Geometry: final body of the model. Coordinates: model frame, mm. Give positions to 0.01 mm unless a question says otherwise; leave off trailing zeros. Loops run counter-clockwise (first coordinate to the right, second up) from the corner with the lowest first, then second, coordinate; pieces in that order, holes last. Notation, with made-up numbers: (7.25, 31.5) -> (13.25, 31.5) arc R11 cw to (13.25, 48.5) -> close; hole circle Ø11 at (75.5, 1.25). An arc over 180 degrees is marked (long way). One line per question, with ' | ' between items. Start each with the question number.
Item 1: Section D-D on x = 35.5. Return loops of the section in (y, z) (3 decimals).
Item 2: Pin query (flat end, axial travel): P1, Ø3, axis at x = 33, y = -23.5, coming from the +Z side. Return the tip coordinate at first contact, or that it passes through.
Item 3: Material intervals for line 1 along Z through (x, y) = (22, -20); line 2 along Y through (x, z) = (26, 43); line 3 along Z through (x, y) = (41, -22), sorted ascending. Write a range as [from, to].
Item 4: Section A-A on x = 7. Return loops of the section in (y, z) (3 decimals), then the cut area to 3 significant figures.
Item 5: Section C-C on x = 26.7. Return loops of the section in (y, z) (3 decimals).
Item 6: Section B-B on z = 22. Return loops of the section in (x, y) (3 decimals).
Item 7: Mould query, pull axis Y, two halves, no side actions, for faces 1 (the flat face through (27, 0, 43.675)), 2 (the flat face through (16, 0, 43.875)), 3 (the cylindrical face through (16.76, -26.67, 41.02)). Classes: released by +Y, released by -Y, zero draft, split by the parting line, or undercut.
from build123d import *

# Parameters (mm, degrees)
SKETCH1_W           = 87.75
SKETCH1_H           = 59.35
BOSS_EXTRUDE1_DEPTH = 43.05
FILLET1_R           = 10
SKETCH2_R           = 4.3
CUT_EXTRUDE1_DEPTH  = 0.2


with BuildPart() as part:
    # Sketch1 → Boss-Extrude1 (new body)
    with BuildSketch(Plane(origin=(0, 0, 0), x_dir=(0, 0, -1), z_dir=(1, 0, 0))):
        Rectangle(SKETCH1_W, SKETCH1_H)
    extrude(amount=BOSS_EXTRUDE1_DEPTH)

    # Fillet1
    fillet1_edges = [part.edges().sort_by_distance(p)[0] for p in [
        (43.05, 0, 43.875),
        (43.05, -29.675, 0),
        (43.05, 0, -43.875),
        (21.525, -29.675, -43.875),
        (21.525, -29.675, 43.875),
        (21.525, 29.675, 43.875),
        (21.525, 29.675, -43.875),
        (43.05, 29.675, 0),
    ]]
    fillet(fillet1_edges, radius=FILLET1_R)

    # Sketch2 → Cut-Extrude1 (cut)
    with BuildSketch(Plane.XY.offset(43.875)):
        with Locations((26.7, 0)):
            Circle(SKETCH2_R)
    extrude(amount=-CUT_EXTRUDE1_DEPTH, mode=Mode.SUBTRACT)


solid = part.part
Result sheet:
1) outline: (-29.37, -33.875) arc R9.695 ccw to (-19.675, -43.57) -> (19.675, -43.57) arc R9.695 ccw to (29.37, -33.875) -> (29.37, 33.875) arc R9.695 ccw to (19.675, 43.57) -> (-19.675, 43.57) arc R9.695 ccw to (-29.37, 33.875) -> close
2) P1: stops at z = 43.6
3) line 1: z = [-43.87, 43.87] | line 2: y = [-23.77, 23.77] | line 3: z = [-39.48, 39.48]
4) outline: (-29.675, -33.875) arc R10 ccw to (-19.675, -43.875) -> (19.675, -43.875) arc R10 ccw to (29.675, -33.875) -> (29.675, 33.875) arc R10 ccw to (19.675, 43.875) -> (-19.675, 43.875) arc R10 ccw to (-29.675, 33.875) -> close | area: 5,120 mm²
5) outline: (-29.675, -33.875) arc R10 ccw to (-19.675, -43.875) -> (19.675, -43.875) arc R10 ccw to (29.675, -33.875) -> (29.675, 33.875) arc R10 ccw to (19.675, 43.875) -> (4.3, 43.875) -> (4.3, 43.675) -> (-4.3, 43.675) -> (-4.3, 43.875) -> (-19.675, 43.875) arc R10 ccw to (-29.675, 33.875) -> close
6) outline: (0, -29.675) -> (33.05, -29.675) arc R10 ccw to (43.05, -19.675) -> (43.05, 19.675) arc R10 ccw to (33.05, 29.675) -> (0, 29.675) -> close
7) face 1: undercut | face 2: zero draft | face 3: released by -Y
